Geometry check sheet. Reference: the model listing, model coordinates, mm. Face numbers are marked on the shaded views. A direction names the side the tool comes from. Coordinates: 2 decimals unless noted, no trailing zeros. Loops run counter-clockwise (first coordinate to the right, second up) from the corner with the lowest first, then second, coordinate; pieces in that order, holes last. Notation, with made-up numbers: (66.25, -29) -> (124.25, -29) arc R17 cw to (124.25, 0) -> close; hole circle Ø1 at (22, 44.25). An arc over 180 degrees is marked (long way). Answer as a JSON object with one key per item and string values.
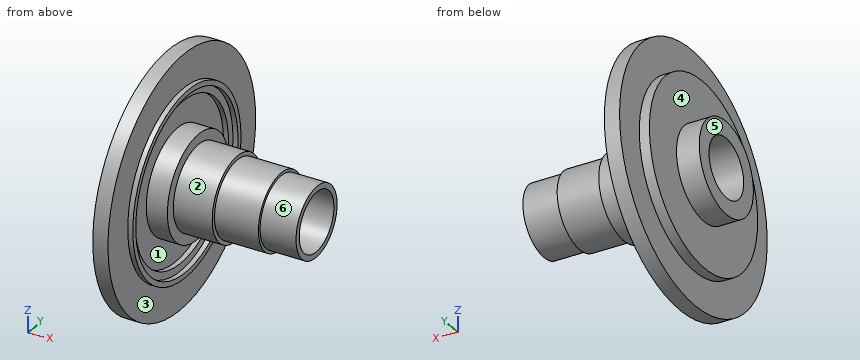
from build123d import *

# Parameters (mm, degrees)
F0_R           = 75
F1_DEPTH       = 9
F2_R           = 54.975
F2_R_2         = 51.975
F3_DEPTH       = 3
F4_R           = 47.5
F5_DEPTH       = 3
F6_R           = 54.975
F7_DEPTH       = 6
F8_R           = 30.975
F9_DEPTH       = 12.5
F10_R          = 24.9
F11_DEPTH      = 23
F12_R          = 22.575
F13_DEPTH      = 26
F14_R          = 20.875
F15_DEPTH      = 21.25
F16_R          = 27.5
F17_DEPTH      = 13.5
F18_R          = 16.825
F19_DEPTH      = 19.501
F19_DEPTH_BACK = 88.751
F20_R          = 17.625
F21_DEPTH      = 122


with BuildPart() as f1:
    # F0 (on Right) → F1 (new body)
    with BuildSketch(Plane.YZ):
        Circle(F0_R)
    extrude(amount=F1_DEPTH)

    # F2 (on face) → F3 (join)
    with BuildSketch(Plane.YZ.offset(9)):
        Circle(F2_R)
        Circle(F2_R_2, mode=Mode.SUBTRACT)
    extrude(amount=F3_DEPTH)

    # F4 (on face) → F5 (cut)
    with BuildSketch(Plane.YZ.offset(9)):
        Circle(F4_R)
    extrude(amount=-F5_DEPTH, mode=Mode.SUBTRACT)

    # F6 (on face) → F7 (join)
    with BuildSketch(Plane(origin=(0, 0, 0), x_dir=(0, -1, 0), z_dir=(-1, 0, 0))):
        Circle(F6_R)
    extrude(amount=F7_DEPTH)

    # F8 (on face) → F9 (join)
    with BuildSketch(Plane.YZ.offset(6)):
        Circle(F8_R)
    extrude(amount=F9_DEPTH)

    # F10 (on face) → F11 (join)
    with BuildSketch(Plane.YZ.offset(18.5)):
        Circle(F10_R)
    extrude(amount=F11_DEPTH)

    # F12 (on face) → F13 (join)
    with BuildSketch(Plane.YZ.offset(41.5)):
        Circle(F12_R)
    extrude(amount=F13_DEPTH)

    # F14 (on face) → F15 (join)
    with BuildSketch(Plane.YZ.offset(67.5)):
        Circle(F14_R)
    extrude(amount=F15_DEPTH)

    # F16 (on face) → F17 (join)
    with BuildSketch(Plane(origin=(-6, 0, 0), x_dir=(0, -1, 0), z_dir=(-1, 0, 0))):
        Circle(F16_R)
    extrude(amount=F17_DEPTH)

    # F18 (on Right) → F19 (cut, two sides)
    with BuildSketch(Plane.YZ) as f19_sk:
        Circle(F18_R)
    extrude(amount=-F19_DEPTH, mode=Mode.SUBTRACT)
    extrude(f19_sk.sketch, amount=-F19_DEPTH_BACK, mode=Mode.SUBTRACT)

    # F20 (on face) → F21 (cut)
    with BuildSketch(Plane.YZ.offset(88.75)):
        Circle(F20_R)
    extrude(amount=-F21_DEPTH, mode=Mode.SUBTRACT)


solid = f1.part
1. Section check A-A, the plane x = 47. Record the boundary of the cut face in (y, z) (3 decimals), then the cut area to 3 significant figures.
Evaluation:
{"outline": "circle Ø45.15 at (0, 0); hole circle Ø35.25 at (0, 0)", "area": "625 mm^2"}
2. Tool access check on the marked faces 4, 5 and 6. Record the directions out of +Z, -Z, +X, -X, +Y, -Y that give a thin tool (end or side, any length) a straight path to the whole face; none if there is none.
Evaluation:
{"face 4": "-X", "face 5": "+Z, -Z, -X, +Y, -Y", "face 6": "+X"}
3. Depth check by flat-ended pin: P1, Ø1, axis at x = 0, y = 16.5, coming from the +Z side; P2, Ø8, axis at x = 20, y = 32, coming from the +Z side; P3, Ø1.5, axis at x = 18.5, z = -12.5, coming from the +Y side; P4, Ø15, axis at y = -10, z = -0.5, coming from the +X side. Enter the tip coordinate at first touch or a pass-through.
Evaluation:
{"P1": "stops at z = 73.27", "P2": "stops at z = 12.61", "P3": "stops at y = 28.66", "P4": "passes through"}
4. Thickness scan on probe 1 along Z at (x, y) = (6.8, 0) (3 decimals); probe 2 along Z at (x, y) = (9.7, 0) (3 decimals); probe 3 along Z at (x, y) = (46, 0) (3 decimals). Record the ranges inside material, lowest first. Write a range as from..to.
Evaluation:
{"probe 1": "z = -75..-47.5, -30.975..-17.625, 17.625..30.975, 47.5..75", "probe 2": "z = -54.975..-51.975, -30.975..-17.625, 17.625..30.975, 51.975..54.975", "probe 3": "z = -22.575..-17.625, 17.625..22.575"}
5. Mould release check, pull along Z, two halves, no side actions. Record for the marked faces 1, 2 and 3: released by +Z, released by -Z, zero draft, split by the parting line, or undercut.
Evaluation:
{"face 1": "undercut", "face 2": "split by the parting line", "face 3": "zero draft"}
